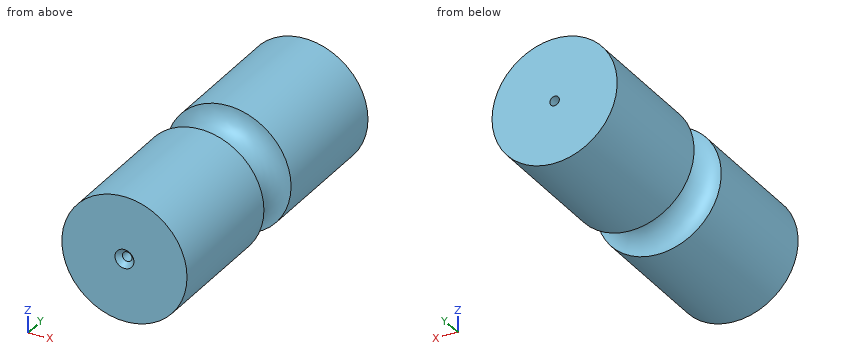
from build123d import *

# Parameters (mm, degrees)
F3_D           = 15.5
F3_CSINK_D     = 30.8
F3_CSINK_ANGLE = 90


with BuildPart() as f1:
    # F0 (on Top) → F1 (revolve)
    with BuildSketch(Plane.XY):
        with BuildLine():
            Line((101.6, 254), (0, 254))
            Line((0, 254), (0, -254))
            Line((0, -254), (101.6, -254))
            Line((101.6, -254), (101.6, -38.1))
            ThreePointArc((101.6, -38.1), (63.5, 0), (101.6, 38.1))
            Line((101.6, 38.1), (101.6, 254))
        make_face()
    revolve(axis=Axis((0, 0, 0), (0, -1, 0)))

    # F3 (through all)
    with Locations(Plane.XZ.offset(254)):
        with Locations((0, 0)):
            CounterSinkHole(F3_D / 2, F3_CSINK_D / 2, counter_sink_angle=F3_CSINK_ANGLE)


solid = f1.part
Model file for the job. Use its own axes, mm. Round coordinates to 2 decimals unless told otherwise and drop trailing zeros. Order: outer loops, then holes, each group sorted by start corner. A loop starts at its lowest first (then second) coordinate and runs counter-clockwise, first axis right, second up.
(1) Band-saw the part on D-D (y = -8.5). List the corners of the cut face in (x, z).
(2) Band-saw the part on B-B (x = 0). List the corners of the cut face in (y, z).
(3) Drill centre lines: line 1 (Y direction, x = 37.5, z = 76.5); line 2 (Y direction, x = -76, z = -25); line 3 (Z direction, x = 1.5, y = -53). Where is each one in solid material? Low to high.
(4) Band-saw the part on C-C (y = 215.5). List the corners of the cut face in (x, z).
(5) Pin check, flat tips, straight feed: pin 1 (2 mm diameter, centred on x = -4, y = -5, fed in from -Z); pin 2 (8 mm diameter, centred on y = -29.5, z = 12.5, fed in from -X); pin 3 (1 mm diameter, centred on x = -53, y = -92.5, fed in from -Z). Stop position of each tip, or through.
(6) Band-saw the part on A-A (z = 0). List the corners of the cut face in (x, y), then the cut area to 3 significant figures.
Verdict:
1. outline: circle Ø128.92 at (0, 0); hole circle Ø15.5 at (0, 0)
2. outline: (-254, -101.6) - (-38.1, -101.6) arc R38.1 cw to (38.1, -101.6) - (254, -101.6) - (254, -7.75) - (-246.35, -7.75) - (-254, -15.4) - close; (-254, 15.4) - (-246.35, 7.75) - (254, 7.75) - (254, 101.6) - (38.1, 101.6) arc R38.1 cw to (-38.1, 101.6) - (-254, 101.6) - close
3. line 1: y = -254 to -34.39, 34.39 to 254
3. line 2: y = -254 to -31.39, 31.39 to 254
3. line 3: z = -101.59 to -7.6, 7.6 to 101.59
4. outline: circle Ø203.2 at (0, 0); hole circle Ø15.5 at (0, 0)
5. pin 1: stops at z = -63.86
5. pin 2: stops at x = -82.53
5. pin 3: stops at z = -86.98
6. outline: (-101.6, -254) - (-15.4, -254) - (-7.75, -246.35) - (-7.75, 254) - (-101.6, 254) - (-101.6, 38.1) arc R38.1 cw to (-101.6, -38.1) - close; (7.75, -246.35) - (15.4, -254) - (101.6, -254) - (101.6, -38.1) arc R38.1 cw to (101.6, 38.1) - (101.6, 254) - (7.75, 254) - close
6. area: 90,700 mm2
